Model file for the job. Use its own axes, mm. Round coordinates to 2 decimals unless told otherwise and drop trailing zeros. Write each loop counter-clockwise with the first axis right and the second up, starting at its lowest first coordinate (ties: lowest second). Pieces come first, ordered by that corner, then holes. Notation, with made-up numbers: (17.25, -38) - (65.25, -38) arc R21 cw to (65.25, -23) - close; hole circle Ø5 at (39.25, 81.5). An arc over 180 degrees is marked (long way). Answer as a JSON object with one key per item and string values. Group by question number.
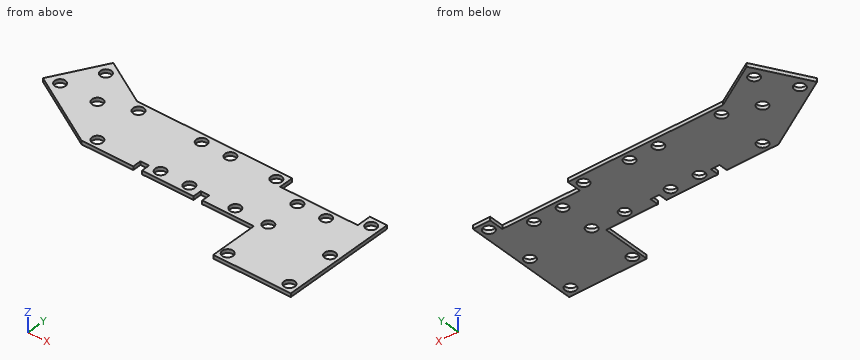
from build123d import *

# Parameters (mm, degrees)
SKETCH1_R           = 4.7625
BOSS_EXTRUDE1_DEPTH = 3.175


with BuildPart() as part:
    # Sketch1 → Boss-Extrude1 (new body)
    with BuildSketch(Plane.XY):
        Polygon((0, 0), (-40.591135768, 23.435303163), (-65.991135768, -20.55878735), (0, -58.65878735), (45.72, -58.65878735), (45.72, -51.03878735), (53.34, -51.03878735), (53.34, -58.65878735), (99.06, -58.65878735), (99.06, -51.03878735), (106.68, -51.03878735), (106.68, -58.65878735), (152.4, -58.65878735), (152.4, -101.6), (220.98, -101.6), (220.98, 0), (205.74, 0), (205.74, -12.7), (137.16, -12.7), (137.16, 0), (99.06, 0), align=None)
        with Locations((-20.295567884, -17.611742094)):
            Circle(SKETCH1_R, mode=Mode.SUBTRACT)
        with Locations((-53.291135768, -17.611742094)):
            Circle(SKETCH1_R, mode=Mode.SUBTRACT)
        with Locations((-36.793351826, 10.963257906)):
            Circle(SKETCH1_R, mode=Mode.SUBTRACT)
        with Locations((7.62, -51.03878735)):
            Circle(SKETCH1_R, mode=Mode.SUBTRACT)
        with Locations((7.62, -7.62)):
            Circle(SKETCH1_R, mode=Mode.SUBTRACT)
        with Locations((63.5, -7.62)):
            Circle(SKETCH1_R, mode=Mode.SUBTRACT)
        with Locations((88.9, -7.62)):
            Circle(SKETCH1_R, mode=Mode.SUBTRACT)
        with Locations((129.54, -7.62)):
            Circle(SKETCH1_R, mode=Mode.SUBTRACT)
        with Locations((88.9, -51.03878735)):
            Circle(SKETCH1_R, mode=Mode.SUBTRACT)
        with Locations((63.5, -51.03878735)):
            Circle(SKETCH1_R, mode=Mode.SUBTRACT)
        with Locations((129.54, -51.03878735)):
            Circle(SKETCH1_R, mode=Mode.SUBTRACT)
        with Locations((158.75, -20.32)):
            Circle(SKETCH1_R, mode=Mode.SUBTRACT)
        with Locations((184.15, -20.32)):
            Circle(SKETCH1_R, mode=Mode.SUBTRACT)
        with Locations((213.36, -7.62)):
            Circle(SKETCH1_R, mode=Mode.SUBTRACT)
        with Locations((213.36, -93.98)):
            Circle(SKETCH1_R, mode=Mode.SUBTRACT)
        with Locations((158.75, -93.98)):
            Circle(SKETCH1_R, mode=Mode.SUBTRACT)
        with Locations((213.36, -51.03878735)):
            Circle(SKETCH1_R, mode=Mode.SUBTRACT)
        with Locations((158.75, -51.03878735)):
            Circle(SKETCH1_R, mode=Mode.SUBTRACT)
    extrude(amount=BOSS_EXTRUDE1_DEPTH)


solid = part.part
(1) Slice it at C-C (x = 213.36). Write the cut outline in (y, z) (1 decimal).
(2) Slice it at A-A (x = 184.15). Write the cut outline in (y, z) (1 decimal).
(3) Slice it at B-B (y = -93.98). Write the cut outline in (x, z) (1 decimal), then the cut area to 3 significant figures.
(4) Slice it at D-D (x = 7.62). Write the cut outline in (y, z) (1 decimal).
(5) Drill centre lines: line 1 (Y direction, x = 129.54, z = 2); line 2 (X direction, y = -95, z = 3); line 3 (X direction, y = -76.5, z = 1.55). Where is each one in solid material? Low to high. Write a range as from..to.
(6) Flat gauge pins, fed straight in: pin 1 (1 mm diameter, centred on x = -4.5, z = 2, fed in from -Y); pin 2 (1 mm diameter, centred on y = -53, z = 1.5, fed in from -X); pin 3 (1 mm diameter, centred on x = 103, z = 1, fed in from -Y). Where does each tip first touch, or does it go through?
Answer:
{
 "1": {"outline": "(-101.6, 0) - (-98.7, 0) - (-98.7, 3.2) - (-101.6, 3.2) - close; (-89.2, 0) - (-55.8, 0) - (-55.8, 3.2) - (-89.2, 3.2) - close; (-46.3, 0) - (-12.4, 0) - (-12.4, 3.2) - (-46.3, 3.2) - close; (-2.9, 0) - (0, 0) - (0, 3.2) - (-2.9, 3.2) - close"},
 "2": {"outline": "(-101.6, 0) - (-25.1, 0) - (-25.1, 3.2) - (-101.6, 3.2) - close; (-15.6, 0) - (-12.7, 0) - (-12.7, 3.2) - (-15.6, 3.2) - close"},
 "3": {"outline": "(152.4, 0) - (154, 0) - (154, 3.2) - (152.4, 3.2) - close; (163.5, 0) - (208.6, 0) - (208.6, 3.2) - (163.5, 3.2) - close; (218.1, 0) - (221, 0) - (221, 3.2) - (218.1, 3.2) - close", "area": "157 mm²"},
 "4": {"outline": "(-58.7, 0) - (-55.8, 0) - (-55.8, 3.2) - (-58.7, 3.2) - close; (-46.3, 0) - (-12.4, 0) - (-12.4, 3.2) - (-46.3, 3.2) - close; (-2.9, 0) - (0, 0) - (0, 3.2) - (-2.9, 3.2) - close"},
 "5": {"line 1": "-58.66..-55.8, -46.28..-12.38, -2.86..0", "line 2": "152.4..154.1, 163.4..208.71, 218.01..220.98", "line 3": "152.4..220.98"},
 "6": {"pin 1": "y = -56.35", "pin 2": "x = -10.67", "pin 3": "y = -51.04"}
}
